Print and shaded views of the part. All mm, measured from the part's lowest x, y and z. Round coordinates to 2 decimals unless told otherwise and drop trailing zeros. Loops run counter-clockwise (first coordinate to the right, second up) from the corner with the lowest first, then second, coordinate; pieces in that order, holes last. Notation, with made-up numbers: (72.25, 1) - (116.25, 1) arc R33 ccw to (116.25, 34) - close; hole circle Ø2 at (1.25, 10.25). An arc over 180 degrees is marked (long way). Answer as a JSON object with one key per item and string values.
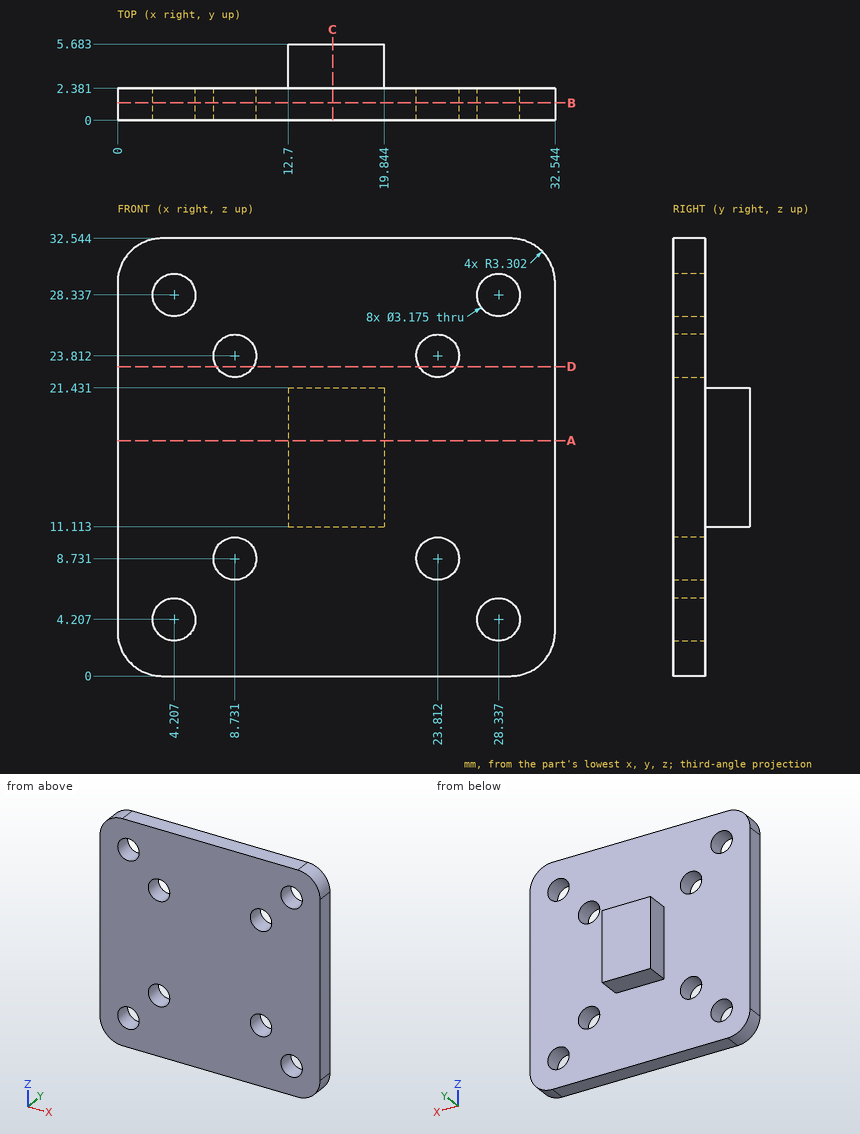
1) Slice it at D-D on z = 23. List the corners of the cut face in (x, y) (1 decimal).
Values follow:
{"outline": "(0, 0) - (7.4, 0) - (7.4, 2.4) - (0, 2.4) - close; (10.1, 0) - (22.4, 0) - (22.4, 2.4) - (10.1, 2.4) - close; (25.2, 0) - (32.5, 0) - (32.5, 2.4) - (25.2, 2.4) - close"}
2) Drop flat-ended pins along their axis: P1, Ø2.5, axis at y = 4, z = 14, coming from the -X side; P2, Ø1.7, axis at x = 15.5, y = 3.5, coming from the -Z side; P3, Ø5, axis at x = 23.81, z = 8.73, coming from the +Y side. Give the stop position or say it passes through.
Values follow:
{"P1": "x = 12.7", "P2": "z = 11.11", "P3": "y = 2.38"}
3) Slice it at B-B on y = 1.3. Count the separate pieces of the cut face and the enclosed holes in it.
Values follow:
{"separate pieces": "1", "enclosed holes": "8"}
4) Slice it at C-C on x = 16. List the corners of the cut face in (y, z).
Values follow:
{"outline": "(0, 0) - (2.38, 0) - (2.38, 11.11) - (5.68, 11.11) - (5.68, 21.43) - (2.38, 21.43) - (2.38, 32.54) - (0, 32.54) - close"}
5) Slice it at A-A on z = 17.5. List the corners of the cut face in (x, y).
Values follow:
{"outline": "(0, 0) - (32.54, 0) - (32.54, 2.38) - (19.84, 2.38) - (19.84, 5.68) - (12.7, 5.68) - (12.7, 2.38) - (0, 2.38) - close"}
6) Probe probe 1 along X at (y, z) = (1.8, 24) (1 decimal); probe 2 along X at (y, z) = (0.25, 29.5) (1 decimal); probe 3 along Z at (x, y) = (5.5, 1.1) (1 decimal). List the from-to ranges inside material, lowest first.
Values follow:
{"probe 1": "0 to 7.2, 10.3 to 22.2, 25.4 to 32.5", "probe 2": "0 to 3.1, 5.3 to 27.3, 29.4 to 32.5", "probe 3": "0 to 3.3, 5.1 to 27.4, 29.3 to 32.5"}
